from build123d import *

# Parameters (mm, degrees)
SCHIZZO1_W                   = 550
SCHIZZO1_H                   = 230
ESTRUSIONE_ESTRUSIONE1_DEPTH = 10
SCHIZZO2_R                   = 2.25
SCHIZZO2_W                   = 66
SCHIZZO2_H                   = 40
TAGLIO_ESTRUSIONE1_DEPTH     = 10


with BuildPart() as part:
    # Schizzo1 → Estrusione-Estrusione1 (new body)
    with BuildSketch(Plane.XY):
        Rectangle(SCHIZZO1_W, SCHIZZO1_H)
    extrude(amount=ESTRUSIONE_ESTRUSIONE1_DEPTH)

    # Schizzo2 → Taglio-Estrusione1 (cut)
    with BuildSketch(Plane(origin=(0, 0, 0), x_dir=(-1, 0, 0), z_dir=(0, 0, -1))):
        with Locations((-217, 91.5)):
            Circle(SCHIZZO2_R)
        with Locations((-217, 73)):
            Circle(SCHIZZO2_R)
        with Locations((217, 91.5)):
            Circle(SCHIZZO2_R)
        with Locations((217, 73)):
            Circle(SCHIZZO2_R)
        with Locations((-257, -107)):
            Circle(SCHIZZO2_R)
        with Locations((257, -107)):
            Circle(SCHIZZO2_R)
        with Locations((132.925688, -84.3)):
            Rectangle(SCHIZZO2_W, SCHIZZO2_H)
    extrude(amount=-TAGLIO_ESTRUSIONE1_DEPTH, mode=Mode.SUBTRACT)


solid = part.part
Check sheet for the modelled part. Datum: model origin and axes. Units: mm. A direction names the side the tool comes from. Give positions to 0.01 mm unless a question says otherwise; leave off trailing zeros. Write each loop counter-clockwise with the first axis right and the second up, starting at its lowest first coordinate (ties: lowest second). Pieces come first, ordered by that corner, then holes. Notation, with made-up numbers: (67.5, 4.5) -> (98.5, 4.5) arc R14 ccw to (98.5, 23.5) -> close; hole circle Ø4 at (47, 13.5). An arc over 180 degrees is marked (long way). Use one line per item in the form item = value. Start each with the question number.
1. Mould release check, pull along Y, two halves, no side actions. Record for faces 3 (the flat face through (-4, 2, 0)), 4 (the flat face through (-132, -104.3, 5)), 5 (the flat face through (-4, -115, 5)): pulls with the +Y half, pulls with the -Y half, needs draft (parallel to the pull), parting line crosses it, or undercut.
2. Access from +Z, -Z, +X, -X, +Y, -Y to the whole of each face (thin tool, end or side, straight path). Record for faces 1 (the flat face through (-4, 2, 10)), 2 (the flat face through (-99.926, -85, 5)).
3. Go/stop test with a flat-tipped pin: P1, Ø4, axis at x = -217, y = 91.5, coming from the -Z side. Record where the tip stops, or that it passes through.
4. Section check B-B (z = 4.75). Record the cut outline in (x, y), and give its area (3 significant figures).
5. Section check A-A (y = -75.5). Record the cut outline in (x, z).
6. Thickness scan on line 1 along Y through (x, z) = (-217, 2.75); line 2 along Y through (x, z) = (257, 4); line 3 along Y through (x, z) = (-121, 8.75). Record the ranges inside material, lowest first. Write a range as from..to.
Conclusion:
q1.face_3 = needs draft
q1.face_4 = undercut
q1.face_5 = pulls with the -Y half
q2.face_1 = +Z, +X, -X, +Y, -Y
q2.face_2 = +Z, -Z
q3.P1 = through
q4.outline = (-275, -115) -> (275, -115) -> (275, 115) -> (-275, 115) -> close; hole circle Ø4.5 at (-257, -107); hole circle Ø4.5 at (-217, 73); hole circle Ø4.5 at (-217, 91.5); hole (-165.93, -104.3) -> (-99.93, -104.3) -> (-99.93, -64.3) -> (-165.93, -64.3) -> close; hole circle Ø4.5 at (217, 73); hole circle Ø4.5 at (217, 91.5); hole circle Ø4.5 at (257, -107)
q4.area = 124,000 mm²
q5.outline = (-275, 0) -> (-165.93, 0) -> (-165.93, 10) -> (-275, 10) -> close; (-99.93, 0) -> (275, 0) -> (275, 10) -> (-99.93, 10) -> close
q6.line_1 = -115..70.75, 75.25..89.25, 93.75..115
q6.line_2 = -115..-109.25, -104.75..115
q6.line_3 = -115..-104.3, -64.3..115
